from build123d import *

# Parameters (mm, degrees)
SKETCH1_W           = 10
SKETCH1_H           = 55.4
SKETCH1_R           = 1.65
SKETCH1_W_2         = 4.5
SKETCH1_H_2         = 10
BOSS_EXTRUDE1_DEPTH = 3


with BuildPart() as part:
    # Sketch1 → Boss-Extrude1 (new body)
    with BuildSketch(Plane(origin=(0, 0, 0), x_dir=(1, 0, 0), z_dir=(0, 1, 0))):
        with Locations((0, -22.7)):
            Rectangle(SKETCH1_W, SKETCH1_H)
        Circle(SKETCH1_R, mode=Mode.SUBTRACT)
        with Locations((-7.25, 0)):
            Rectangle(SKETCH1_W_2, SKETCH1_H_2)
        with Locations((7.25, 0)):
            Rectangle(SKETCH1_W_2, SKETCH1_H_2)
    extrude(amount=BOSS_EXTRUDE1_DEPTH)


solid = part.part
Input: part model. Units: mm. Frame: model coordinates. A direction names the side the tool comes from. Give positions to 0.01 mm unless a question says otherwise; leave off trailing zeros. Order: outer loops, then holes, each group sorted by start corner. A loop starts at its lowest first (then second) coordinate and runs counter-clockwise, first axis right, second up.
Q1. Section C-C on z = 0. Output: boundary loops of the cut face in (x, y).
Checked values:
outline: (-9.5, 0) - (-1.65, 0) - (-1.65, 3) - (-9.5, 3) - close; (1.65, 0) - (9.5, 0) - (9.5, 3) - (1.65, 3) - close
Q2. Section B-B on y = 2.35. Output: boundary loops of the cut face in (x, z).
Checked values:
outline: (-9.5, -5) - (9.5, -5) - (9.5, 5) - (5, 5) - (5, 50.4) - (-5, 50.4) - (-5, 5) - (-9.5, 5) - close; hole circle Ø3.3 at (0, 0)
Q3. Section A-A on x = 0. Output: boundary loops of the cut face in (y, z).
Checked values:
outline: (0, -5) - (3, -5) - (3, -1.65) - (0, -1.65) - close; (0, 1.65) - (3, 1.65) - (3, 50.4) - (0, 50.4) - close
Q4. Section D-D on z = 43. Output: boundary loops of the cut face in (x, y), and give its area (3 significant figures).
Checked values:
outline: (-5, 0) - (5, 0) - (5, 3) - (-5, 3) - close
area: 30.0 mm2
Q5. Draft query along Z for faces 1 (the flat face through (-9.5, 1, 0)), 2 (the cylindrical face through (-1.216, 1.479, -1.115)), 3 (the flat face through (0, 1, 50.4)). Return one class per face: +Z half, -Z half, draft (parallel to the pull), parting line (faces both ways), or undercut.
Checked values:
face 1: draft
face 2: undercut
face 3: +Z half
Q6. Set-up query: faces 4 (the flat face through (-5, 1, 28)), 5 (the flat face through (9.5, 1, 0)), 6 (the flat face through (5, 1, 28)). Return all of +Z, -Z, +X, -X, +Y, -Y with unobstructed straight access to the full face (end or side cutting, diameter ignored); none if empty.
Checked values:
face 4: +Z, -X, +Y, -Y
face 5: +Z, -Z, +X, +Y, -Y
face 6: +Z, +X, +Y, -Y
Q7. Ray query, probe 1 along X at (y, z) = (1.2, 0); probe 2 along Z at (x, y) = (0, 1.4); probe 3 along X at (y, z) = (1.6, 14.5). Return the intervals inside material, ascending.
Checked values:
probe 1: x = -9.5 to -1.65, 1.65 to 9.5
probe 2: z = -5 to -1.65, 1.65 to 50.4
probe 3: x = -5 to 5
Q8. Contact query for flat-ended pins moving along their axis: pin 1 Ø0.9 at (y, z) = (2, 20) entering from +X; pin 2 Ø1.5 at (x, z) = (-4.5, 30.5) entering from -Y; pin 3 Ø1.5 at (x, y) = (-7.5, 1) entering from +Z. Output: stop coordinate, or through.
Checked values:
pin 1: stops at x = 5
pin 2: stops at y = 0
pin 3: stops at z = 5
